```python
from build123d import *

# Parameters (mm, degrees)
SKETCH1_R           = 1.5
SKETCH1_R_2         = 11
BOSS_EXTRUDE1_DEPTH = 20
SKETCH1_3_R         = 1.5
BOSS_EXTRUDE2_DEPTH = 17.5


with BuildPart() as part:
    # Sketch1 → Boss-Extrude1 (new body)
    with BuildSketch(Plane(origin=(0, 0, 0), x_dir=(1, 0, 0), z_dir=(0, 1, 0))):
        Polygon((-15.493145751, 21.15), (-21.15, 15.493145751), (-21.15, -15.493145751), (-15.493145751, -21.15), (15.493145751, -21.15), (21.15, -15.493145751), (21.15, 15.493145751), (15.493145751, 21.15), (12, 21.15), (-12, 21.15), align=None)
        with Locations(Location((-15.5, -15.5, 0), (0, 0, 270))):
            Circle(SKETCH1_R, mode=Mode.SUBTRACT)
        with Locations(Location((15.5, -15.5, 0), (0, 0, 270))):
            Circle(SKETCH1_R, mode=Mode.SUBTRACT)
        with Locations(Location((0, 0, 0), (0, 0, 270))):
            Circle(SKETCH1_R_2, mode=Mode.SUBTRACT)
        with Locations(Location((-15.5, 15.5, 0), (0, 0, 270))):
            Circle(SKETCH1_R, mode=Mode.SUBTRACT)
        with Locations(Location((15.5, 15.5, 0), (0, 0, 270))):
            Circle(SKETCH1_R, mode=Mode.SUBTRACT)
    extrude(amount=BOSS_EXTRUDE1_DEPTH)

    # Sketch1<3> → Boss-Extrude2 (add)
    with BuildSketch(Plane(origin=(0, 0, 0), x_dir=(1, 0, 0), z_dir=(0, 1, 0))):
        with Locations(Location((15.5, -15.5, 0), (0, 0, 270))):
            Circle(SKETCH1_3_R)
        with Locations(Location((-15.5, -15.5, 0), (0, 0, 270))):
            Circle(SKETCH1_3_R)
        with Locations(Location((15.5, 15.5, 0), (0, 0, 270))):
            Circle(SKETCH1_3_R)
        with Locations(Location((-15.5, 15.5, 0), (0, 0, 270))):
            Circle(SKETCH1_3_R)
    extrude(amount=BOSS_EXTRUDE2_DEPTH)


solid = part.part
```
Here's how the part is built. I have some questions about the finished solid (model axes, mm). A direction names the side the tool comes from. Coordinates: 2 decimals unless noted, no trailing zeros. Order: outer loops, then holes, each group sorted by start corner. A loop starts at its lowest first (then second) coordinate and runs counter-clockwise, first axis right, second up.
1) We'd pull the mould along Z, two halves only. Please class faces 3 (the face through (16, 17.5, -16)), 4 (the face through (0, 10, 21.15)), 5 (the face through (-15, 17.5, -16)), 6 (the face through (0, 10, -21.15)): +Z half, -Z half, draft (parallel to the pull), parting line (faces both ways), or undercut.
2) Imagine slicing it at D-D on y = 18.75. List the corners of the cut face in (x, z) for me, and give its area (3 significant figures).
3) Imagine slicing it at A-A on x = 0. List the corners of the cut face in (y, z) for me, and give its area (3 significant figures).
4) Which directions (+Z, -Z, +X, -X, +Y, -Y) give clear straight access to the entire face, cutting with the end or side of a thin tool? Please do faces 1 (the face through (-10.74, 9.86, -2.38)), 2 (the face through (16, 17.5, 15)).
5) Imagine slicing it at C-C on y = 9.25. List the corners of the cut face in (x, z) for me.
6) Imagine slicing it at B-B on z = 0. List the corners of the cut face in (x, y) for me, and give its area (3 significant figures).
7) Will this pin go through, and if not, where does the flat tip stop? pin 1 (1.5 mm diameter, centred on x = -15.5, z = 16, fed in from +Y).
8) I need wall thicknesses on line 1 (X direction, y = 19.25, z = -15.5); line 2 (X direction, y = 6.75, z = 0); line 3 (X direction, y = 5.25, z = -7). Which ranges of each line are inside material? Lowest first, please.
Response values:
1. face 3: undercut
1. face 4: +Z half
1. face 5: undercut
1. face 6: -Z half
2. outline: (-21.15, -15.49) - (-15.49, -21.15) - (15.49, -21.15) - (21.15, -15.49) - (21.15, 15.49) - (15.49, 21.15) - (-15.49, 21.15) - (-21.15, 15.49) - close; hole circle Ø3 at (-15.5, -15.5); hole circle Ø3 at (-15.5, 15.5); hole circle Ø22 at (0, 0); hole circle Ø3 at (15.5, -15.5); hole circle Ø3 at (15.5, 15.5)
2. area: 1,320 mm2
3. outline: (0, -21.15) - (20, -21.15) - (20, -11) - (0, -11) - close; (0, 11) - (20, 11) - (20, 21.15) - (0, 21.15) - close
3. area: 406 mm2
4. face 1: +Y, -Y
4. face 2: +Y
5. outline: (-21.15, -15.49) - (-15.49, -21.15) - (15.49, -21.15) - (21.15, -15.49) - (21.15, 15.49) - (15.49, 21.15) - (-15.49, 21.15) - (-21.15, 15.49) - close; hole circle Ø22 at (0, 0)
6. outline: (-21.15, 0) - (-11, 0) - (-11, 20) - (-21.15, 20) - close; (11, 0) - (21.15, 0) - (21.15, 20) - (11, 20) - close
6. area: 406 mm2
7. pin 1: stops at y = 17.5
8. line 1: x = -21.14 to -17, -14 to 14, 17 to 21.14
8. line 2: x = -21.15 to -11, 11 to 21.15
8. line 3: x = -21.15 to -8.49, 8.49 to 21.15
